```python
from build123d import *

# Parameters (mm, degrees)
CROQUIS3_R               = 7.5
SALIENTE_EXTRUIR10_DEPTH = 7.5
SALIENTE_EXTRUIR24_DEPTH = 7.5
CROQUIS5_R               = 6.3
CORTAR_EXTRUIR1_DEPTH    = 10
MATRIZC1_COUNT           = 3
MATRIZC2_START           = -8.85913735
MATRIZC2_OUTLINE_R       = 6.3
MATRIZC2_DEPTH           = 15
MATRIZC2_START_2         = -6.14086265
MATRIZC2_2_OUTLINE_R     = 6.3
MATRIZC2_2_DEPTH         = 15
MATRIZC3_COUNT           = 3


# Read off the part's stored shape, not the designer's step: MatrizC2
with BuildPart() as part:
    # Croquis1 → Revolución1 (revolve)
    with BuildSketch(Plane(origin=(0, 0, 0), x_dir=(0, 0, -1), z_dir=(1, 0, 0)), mode=Mode.PRIVATE) as revoluci_n1_sk:
        Polygon((0, 90), (0, -125), (17.5, -125), (17.5, -75), (22.5, -75), (22.5, 75), (46.2, 75), (46.2, 90), align=None)
    revolve(revoluci_n1_sk.sketch.rotate(Axis((0, 90, 0), (0, -1, 0)), 180), axis=Axis((0, 90, 0), (0, -1, 0)))

    # Croquis3 → Saliente-Extruir10 (add, symmetric)
    with BuildSketch(Plane(origin=(0, 0, 0), x_dir=(0, 0, -1), z_dir=(1, 0, 0))):
        with BuildLine():
            Line((-22.5, 90), (19.926406871, 90))
            Line((19.926406871, 90), (83.566017178, 153.639610307))
            ThreePointArc((83.566017178, 153.639610307), (83.566017178, 174.852813742), (62.352813742, 174.852813742))
            Line((62.352813742, 174.852813742), (-22.5, 90))
        make_face()
        with Locations((72.95941546, 164.246212025)):
            Circle(CROQUIS3_R, mode=Mode.SUBTRACT)
    saliente_extruir10 = extrude(amount=SALIENTE_EXTRUIR10_DEPTH, both=True)

    # Croquis4 → Saliente-Extruir24 (add, symmetric)
    with BuildSketch(Plane(origin=(0, 0, 0), x_dir=(0, 0, -1), z_dir=(1, 0, 0))):
        with BuildLine():
            Line((-22.5, -75), (-111.800673807, -164.399250863))
            ThreePointArc((-111.800673807, -164.399250863), (-112.093769258, -185.298983205), (-91.211457576, -186.201078383))
            Line((-91.211457576, -186.201078383), (-22.5, -125))
            Line((-22.5, -125), (-3.021288489, -125))
            Line((-3.021288489, -125), (-3.021288489, -75))
            Line((-3.021288489, -75), (-22.5, -75))
        make_face()
    saliente_extruir24 = extrude(amount=SALIENTE_EXTRUIR24_DEPTH, both=True)

    # Croquis5 → Cortar-Extruir1 (cut, symmetric)
    with BuildSketch(Plane(origin=(0, 0, 0), x_dir=(0, 0, -1), z_dir=(1, 0, 0))):
        with Locations((-101.188222736, -175)):
            Circle(CROQUIS5_R)
    extrude(amount=CORTAR_EXTRUIR1_DEPTH, both=True, mode=Mode.SUBTRACT)

    # MatrizC1: Saliente-Extruir24 ×3 about axis
    matrizc1_axis = Axis((0, 0, 1.56939663), (0, 1, 0))
    for i in range(1, MATRIZC1_COUNT):
        add(saliente_extruir24.rotate(matrizc1_axis, i * 360 / MATRIZC1_COUNT))

    # MatrizC2 outline → MatrizC2 (cut)
    with BuildSketch(Plane(origin=(0, 0, 0), x_dir=(0.8660254037844362, 0, 0.5000000000000042), z_dir=(0.5000000000000042, 0, -0.8660254037844363)).offset(MATRIZC2_START)):
        with Locations((-100.01457544, 175)):
            Circle(MATRIZC2_OUTLINE_R)
    extrude(amount=MATRIZC2_DEPTH, mode=Mode.SUBTRACT)

    # MatrizC2 2 outline → MatrizC2 2 (cut)
    with BuildSketch(Plane(origin=(0, 0, 0), x_dir=(0.8660254037844431, 0, -0.4999999999999921), z_dir=(0.4999999999999921, 0, 0.8660254037844433)).offset(MATRIZC2_START_2)):
        with Locations((100.01457544, -175)):
            Circle(MATRIZC2_2_OUTLINE_R)
    extrude(amount=MATRIZC2_2_DEPTH, mode=Mode.SUBTRACT)

    # MatrizC3: Saliente-Extruir10 ×3 about axis
    matrizc3_axis = Axis((0, 0, 0.782431531), (0, 1, 0))
    for i in range(1, MATRIZC3_COUNT):
        add(saliente_extruir10.rotate(matrizc3_axis, i * 360 / MATRIZC3_COUNT))


solid = part.part
```
Geometry check sheet. Reference: the model listing, model coordinates, mm. A direction names the side the tool comes from. Coordinates: 2 decimals unless noted, no trailing zeros. Order: outer loops, then holes, each group sorted by start corner. A loop starts at its lowest first (then second) coordinate and runs counter-clockwise, first axis right, second up. Notation, with made-up numbers: M 6.5,36.5 L 21.5,36.5 A25 cw 21.5,64.5 Z; hole C -0.5,84.5 d9. An arc over 180 degrees is marked long. One line per question, with ' | ' between items. Start each with the question number.
Item 1: Gauge pin test, flat ends, axial feed: pin 1 (1.4 mm diameter, centred on x = -3.5, z = 21.5, fed in from +Y); pin 2 (5 mm diameter, centred on x = -4.5, y = -39.5, fed in from -Z); pin 3 (1 mm diameter, centred on y = -70.5, z = 17.5, fed in from +X). Record the tip position at first contact, or that the pin passes through.
Item 2: Cross-section at A-A on y = -175. Enter the section's corners in (x, z).
Item 3: Material ranges on L1, parallel to Z at x = 2, y = -30.5; L2, parallel to Y at x = 17, z = 39; L3, parallel to X at y = -166, z = -29, recorded low to high. Write a range as [from, to].
Item 4: Cross-section at C-C on y = -26. Enter the section's corners in (x, z).
Item 5: Cross-section at D-D on z = 81.5. Enter the section's corners in (x, y), then the cut area to 3 significant figures.
Item 6: Set-up check for faces 4 (the flat face through (-56.306, -119.074, -30.818)), 5 (the flat face through (-48.35, -156.03, -26.22)), 6 (the flat face through (0.1, 95.2, 17.3)), 7 (the flat face through (-7, -75, -17)), 8 (the flat face through (-60.85, -131.7, -24.9)): record each of +Z, -Z, +X, -X, +Y, -Y from which the full face is reachable in a straight line by a thin tool's end or side.
Item 7: Draft check along Y on faces 1 (the flat face through (7.5, -132, 67)), 2 (the flat face through (-14.384, 95.169, -7.401)), 3 (the cylindrical face through (-0.105, 156.925, -71.334)). Enter one of: pulls with the +Y half, pulls with the -Y half, needs draft (parallel to the pull), parting line crosses it, or undercut.
Item 8: Cross-section at B-B on x = -31. Enter the section's corners in (y, z).
Findings:
1) pin 1: stops at y = 91.7 | pin 2: stops at z = -22.41 | pin 3: stops at x = 14.74
2) outline: M -103.01,-49.24 L -95.51,-62.24 L -89,-58.48 L -96.5,-45.49 Z; M -85.59,-39.19 L -78.09,-52.18 L -62.99,-43.46 L -70.49,-30.47 Z; M -7.5,78.64 L 7.5,78.64 L 7.5,94.89 L -7.5,94.89 Z; M -7.5,107.49 L 7.5,107.49 L 7.5,116.19 L -7.5,116.19 Z; M 62.99,-43.46 L 78.09,-52.18 L 85.59,-39.19 L 70.49,-30.47 Z; M 89,-58.48 L 95.51,-62.24 L 103.01,-49.24 L 96.5,-45.49 Z
3) L1: z = [-22.41, 22.41] | L2: y = [75, 90] | L3: x = [-67.95, -59.67], [59.67, 67.95]
4) outline: C 0,0 d45
5) outline: M -7.5,-177.55 L 7.5,-177.55 L 7.5,-134.07 L -7.5,-134.07 Z | area: 652 mm²
6) face 4: -Z, -X | face 5: +Z, -Y | face 6: +Z, +Y | face 7: none | face 8: +Z, -X, -Y
7) face 1: needs draft | face 2: pulls with the +Y half | face 3: undercut
8) outline: M -142.1,-24.99 L -94.22,-24.99 L -85.55,-7.67 L -134.38,-7.67 Z; M 75,-34.26 L 90,-34.26 L 90,34.26 L 75,34.26 Z; M 100.76,10.02 L 143.18,10.02 L 151.84,27.34 L 109.42,27.34 Z
